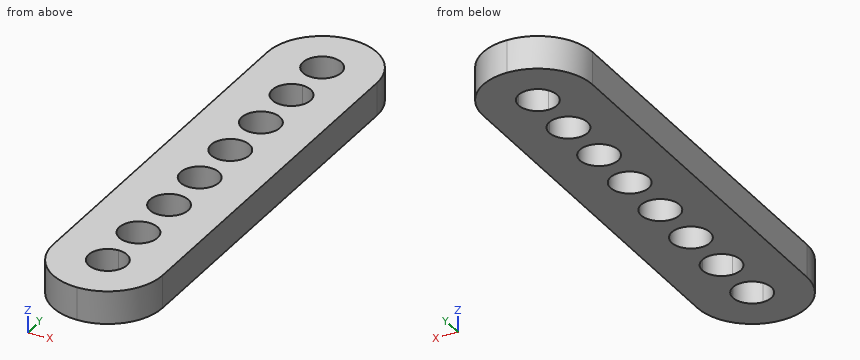
from build123d import *

# Parameters (mm, degrees)
F0_R     = 1.75
F1_DEPTH = 3
F2_R     = 4.99999


# Not quite as in the source:
# - a fillet or chamfer is up to 0.001 mm smaller than in the source, because OpenCascade refuses the exact size


with BuildPart() as f1:
    # F0 (on Top) → F1 (new body)
    with BuildSketch(Plane.XY):
        Polygon((-16.2647291371, -19.261389355), (-16.2647291371, 20.738610645), (-16.2647291371, 25.738610645), (-26.2647291371, 25.738610645), (-26.2647291371, 3.238610645), (-26.2647291371, -19.261389355), (-21.2647291371, -19.261389355), align=None)
        with BuildLine():
            ThreePointArc((-19.5147291371, -14.261389355), (-20.0272922701, -15.4988262221), (-21.2647291371, -16.011389355))
            ThreePointArc((-21.2647291371, -16.011389355), (-23.0147291371, -14.261389355), (-21.2647291371, -12.511389355))
            ThreePointArc((-21.2647291371, -12.511389355), (-20.0272922701, -13.0239524879), (-19.5147291371, -14.261389355))
        make_face(mode=Mode.SUBTRACT)
        with BuildLine():
            ThreePointArc((-19.5147291371, -9.261389355), (-20.0272922701, -10.4988262221), (-21.2647291371, -11.011389355))
            ThreePointArc((-21.2647291371, -11.011389355), (-22.5021660042, -8.0239524879), (-19.5147291371, -9.261389355))
        make_face(mode=Mode.SUBTRACT)
        with Locations((-21.2647291371, -4.261389355)):
            Circle(F0_R, mode=Mode.SUBTRACT)
        with Locations((-21.2647291371, 0.738610645)):
            Circle(F0_R, mode=Mode.SUBTRACT)
        with Locations((-21.2647291371, 5.738610645)):
            Circle(F0_R, mode=Mode.SUBTRACT)
        with Locations((-21.2647291371, 10.738610645)):
            Circle(F0_R, mode=Mode.SUBTRACT)
        with BuildLine():
            ThreePointArc((-19.5147291371, 15.738610645), (-22.5021660042, 14.5011737779), (-21.2647291371, 17.488610645))
            ThreePointArc((-21.2647291371, 17.488610645), (-20.0272922701, 16.9760475121), (-19.5147291371, 15.738610645))
        make_face(mode=Mode.SUBTRACT)
        with BuildLine():
            ThreePointArc((-19.5147291371, 20.738610645), (-20.0272922701, 19.5011737779), (-21.2647291371, 18.988610645))
            ThreePointArc((-21.2647291371, 18.988610645), (-22.5021660042, 21.9760475121), (-19.5147291371, 20.738610645))
        make_face(mode=Mode.SUBTRACT)
    extrude(amount=F1_DEPTH)

    # F2 (radius 5 in the source; OpenCascade refuses exactly that, so slightly less here)
    f2_edges = [f1.edges().sort_by_distance(p)[0] for p in [
        (-16.264729, 25.738611, 1.5),
        (-26.264729, 25.738611, 1.5),
        (-16.264729, -19.261389, 1.5),
        (-26.264729, -19.261389, 1.5),
    ]]
    fillet(f2_edges, radius=F2_R)


solid = f1.part
Model file for the job. Use its own axes, mm. Round coordinates to 2 decimals unless told otherwise and drop trailing zeros. Loops run counter-clockwise (first coordinate to the right, second up) from the corner with the lowest first, then second, coordinate; pieces in that order, holes last.
1. Band-saw the part on B-B, the plane z = 0.6. Count the separate pieces of the cut face and the enclosed holes in it, and give its area (3 significant figures).
Check values:
separate pieces: 1
enclosed holes: 8
area: 352 mm2
2. Band-saw the part on C-C, the plane x = -24.75. List the corners of the cut face in (y, z).
Check values:
outline: (-17.85, 0) - (24.32, 0) - (24.32, 3) - (-17.85, 3) - close
3. Band-saw the part on A-A, the plane y = 9.5. List the corners of the cut face in (x, z), and give its area (3 significant figures).
Check values:
outline: (-26.26, 0) - (-22.5, 0) - (-22.5, 3) - (-26.26, 3) - close; (-20.03, 0) - (-16.26, 0) - (-16.26, 3) - (-20.03, 3) - close
area: 22.6 mm2
4. Wall check: probe 1 along X at (y, z) = (0, 1.2); probe 2 along X at (y, z) = (-9.5, 0.4); probe 3 along Y at (x, z) = (-23.25, 1.6). Give the ranges that are in metal, low to high.
Check values:
probe 1: x = -26.26 to -22.85, -19.68 to -16.26
probe 2: x = -26.26 to -23, -19.53 to -16.26
probe 3: y = -18.85 to 25.33
